```python
from build123d import *

# Parameters (mm, degrees)
SKETCH1_W           = 15
SKETCH1_H           = 20
BOSS_EXTRUDE2_DEPTH = 3
SKETCH2_R           = 3.5
BOSS_EXTRUDE3_DEPTH = 2.5


with BuildPart() as part:
    # Sketch1 → Boss-Extrude2 (new body)
    with BuildSketch(Plane.XY):
        Rectangle(SKETCH1_W, SKETCH1_H)
    extrude(amount=BOSS_EXTRUDE2_DEPTH)

    # Sketch2 → Boss-Extrude3 (add, symmetric)
    with BuildSketch(Plane(origin=(0, 0, 0), x_dir=(1, 0, 0), z_dir=(0, 1, 0))):
        with BuildLine():
            Line((-5, -3), (5, -3))
            Line((5, -3), (5, -12.5))
            ThreePointArc((5, -12.5), (0, -17.5), (-5, -12.5))
            Line((-5, -12.5), (-5, -3))
        make_face()
        with Locations(Location((0, -12.5, 0), (0, 0, 270))):
            Circle(SKETCH2_R, mode=Mode.SUBTRACT)
    extrude(amount=BOSS_EXTRUDE3_DEPTH, both=True)


solid = part.part
```
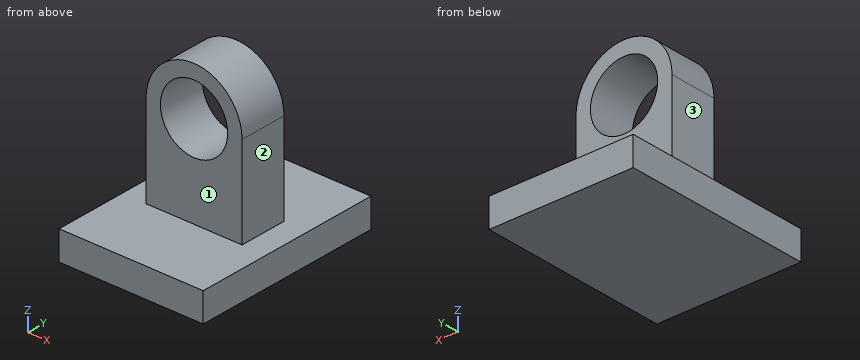
Source: CAD feature listing. Evaluate the final solid. Frame: model axes, mm. Face numbers are marked on the shaded views. A direction names the side the tool comes from. Round coordinates to 2 decimals unless told otherwise and drop trailing zeros. Loops run counter-clockwise (first coordinate to the right, second up) from the corner with the lowest first, then second, coordinate; pieces in that order, holes last. Notation, with made-up numbers: M 45.25,67.25 L 76.25,67.25 A7 cw 76.25,76.25 Z; hole C 33,-32.5 d2. An arc over 180 degrees is marked long. Put each result on its own line as item: value.
(1) Section D-D, the plane x = -3.75. Return loops of the section in (y, z), and give its area (3 significant figures).
Solutions:
outline: M -10,0 L 10,0 L 10,3 L 2.5,3 L 2.5,15.81 L -2.5,15.81 L -2.5,3 L -10,3 Z
area: 124 mm²
(2) Section A-A, the plane x = 0. Return loops of the section in (y, z).
Solutions:
outline: M -10,0 L 10,0 L 10,3 L 2.5,3 L 2.5,9 L -2.5,9 L -2.5,3 L -10,3 Z; M -2.5,16 L 2.5,16 L 2.5,17.5 L -2.5,17.5 Z
(3) First-contact query: pin 1 (6 mm diameter, centred on x = 5.5, z = 14, fed in from +Y); pin 2 (8 mm diameter, centred on y = -3.5, z = 10.5, fed in from +X); pin 3 (2.5 mm diameter, centred on y = -0.5, z = 9, fed in from -X). Flat tips, straight axial feed; report the tip coordinate or a pass-through.
Solutions:
pin 1: y = 2.5
pin 2: x = 5
pin 3: x = -5
(4) Section B-B, the plane z = 15.25. Return loops of the section in (x, y), and give its area (3 significant figures).
Solutions:
outline: M -4.18,-2.5 L -2.17,-2.5 L -2.17,2.5 L -4.18,2.5 Z; M 2.17,-2.5 L 4.18,-2.5 L 4.18,2.5 L 2.17,2.5 Z
area: 20.1 mm²
(5) Ray query, line 1 (X direction, y = 1, z = 12.5); line 2 (Z direction, x = 5.5, y = 6.75); line 3 (Y direction, x = 3, z = 7.5). Return the intervals inside material, ascending. Write a range as [from, to].
Solutions:
line 1: [-5, -3.5], [3.5, 5]
line 2: [0, 3]
line 3: [-2.5, 2.5]
(6) Access query for the marked faces 1, 2 and 3. Directions: +Z, -Z, +X, -X, +Y, -Y. A direction counts if a zero-diameter tool reaches every point of the face in a straight line with its end or side. Return the directions, or none.
Solutions:
face 1: +Z, +X, -X, -Y
face 2: +Z, +X, +Y, -Y
face 3: +Z, -X, +Y, -Y
(7) Section C-C, the plane y = 2. Return loops of the section in (x, z), and give its area (3 significant figures).
Solutions:
outline: M -7.5,0 L 7.5,0 L 7.5,3 L 5,3 L 5,12.5 A5 ccw -5,12.5 L -5,3 L -7.5,3 Z; hole C 0,12.5 d7
area: 141 mm²
